from build123d import *

# Parameters (mm, degrees)
SKETCH_1_R          = 26
SKETCH_1_R_2        = 20
EXTRUDE_1_DEPTH     = 7
SKETCH_2_R          = 23.9
SKETCH_2_R_2        = 22.1
CUT_EXTRUDE_1_DEPTH = 1.5


with BuildPart() as part:
    # 草图1 → 凸台-拉伸1 (new body)
    with BuildSketch(Plane(origin=(0, 0, 0), x_dir=(1, 0, 0), z_dir=(0, 1, 0))):
        Circle(SKETCH_1_R)
        Circle(SKETCH_1_R_2, mode=Mode.SUBTRACT)
    extrude(amount=EXTRUDE_1_DEPTH)

    # 草图2 → 切除-拉伸1 (cut)
    with BuildSketch(Plane(origin=(0, 7, 0), x_dir=(1, 0, 0), z_dir=(0, 1, 0))):
        Circle(SKETCH_2_R)
        Circle(SKETCH_2_R_2, mode=Mode.SUBTRACT)
    cut_extrude_1 = extrude(amount=-CUT_EXTRUDE_1_DEPTH, mode=Mode.SUBTRACT)

    # 镜向1: 切除-拉伸1 across plane
    add(cut_extrude_1.mirror(Plane.ZX.offset(3.5)), mode=Mode.SUBTRACT)


solid = part.part
Could you check a few things on this model? Use its own coordinates, in mm. A direction names the side the tool comes from. Give positions to 0.01 mm unless a question says otherwise; leave off trailing zeros. Order: outer loops, then holes, each group sorted by start corner. A loop starts at its lowest first (then second) coordinate and runs counter-clockwise, first axis right, second up. Notation, with made-up numbers: M -25,26.5 L 16,26.5 A8 cw 16,32.5 Z; hole C -17,7 d8. An arc over 180 degrees is marked long. One line per question, with ' | ' between items.
1. For faces 1 (the face through (12.85, 6.26, -20.15)), 2 (the face through (-4.791, 0.74, 21.574)), 3 (the face through (-4.336, 3.451, 19.524)), which set-ups out of +Z, -Z, +X, -X, +Y, -Y let a thin tool reach every point of the face, with its end or its side?
Results:
face 1: +Y | face 2: -Y | face 3: +Y, -Y
2. I want a section at A-A (z = 0). List the corners of the cut face in (x, y) for me, and give its area (3 significant figures).
Results:
outline: M -26,0 L -23.9,0 L -23.9,1.5 L -22.1,1.5 L -22.1,0 L -20,0 L -20,7 L -22.1,7 L -22.1,5.5 L -23.9,5.5 L -23.9,7 L -26,7 Z; M 20,0 L 22.1,0 L 22.1,1.5 L 23.9,1.5 L 23.9,0 L 26,0 L 26,7 L 23.9,7 L 23.9,5.5 L 22.1,5.5 L 22.1,7 L 20,7 Z | area: 73.2 mm²
3. We'd pull the mould along Z, two halves only. Please class faces 4 (the face through (-5, 0, 20)), 5 (the face through (6.97, 5.5, 21.133)), 6 (the face through (-20.633, 3.451, 15.821)): +Z half, -Z half, draft (parallel to the pull), parting line (faces both ways), or undercut.
Results:
face 4: draft | face 5: undercut | face 6: parting line
4. If I drill on line 1 (Z direction, x = 0, y = 6.1); line 2 (Z direction, x = 0, y = 5), over which ranges is the centre line in solid material (lowest first)?
Results:
line 1: -26 to -23.9, -22.1 to -20, 20 to 22.1, 23.9 to 26 | line 2: -26 to -20, 20 to 26
5. I want a section at B-B (x = 0). List the corners of the cut face in (y, z) for me, and give its area (3 significant figures).
Results:
outline: M 0,-26 L 7,-26 L 7,-23.9 L 5.5,-23.9 L 5.5,-22.1 L 7,-22.1 L 7,-20 L 0,-20 L 0,-22.1 L 1.5,-22.1 L 1.5,-23.9 L 0,-23.9 Z; M 0,20 L 7,20 L 7,22.1 L 5.5,22.1 L 5.5,23.9 L 7,23.9 L 7,26 L 0,26 L 0,23.9 L 1.5,23.9 L 1.5,22.1 L 0,22.1 Z | area: 73.2 mm²
6. I want a section at C-C (y = 4). List the corners of the cut face in (x, z) for me, and give its area (3 significant figures).
Results:
outline: C 0,0 d52; hole C 0,0 d40 | area: 867 mm²
7. I'm going to push flat-ended pins straight in: pin 1 (1.5 mm diameter, centred on x = 10, y = 5, fed in from -Z); pin 2 (4 mm diameter, centred on x = -18, y = 1, fed in from -Z); pin 3 (3 mm diameter, centred on x = -4, y = 1, fed in from -Z); pin 4 (1 mm diameter, centred on x = 15, z = -14.5, fed in from -Y). Where does each tip first touch, or does it pass through?
Results:
pin 1: z = -24.3 | pin 2: z = -20.49 | pin 3: z = -25.88 | pin 4: y = 0
